Verification items for this drawing (mm, ordinates from the low corner). Round coordinates to 2 decimals unless told otherwise and drop trailing zeros. Write each loop counter-clockwise with the first axis right and the second up, starting at its lowest first coordinate (ties: lowest second). Pieces come first, ordered by that corner, then holes. Notation, with made-up numbers: (61, 12) -> (86, 12) arc R10 cw to (86, 26) -> close; hole circle Ø8 at (3.5, 79). An arc over 180 degrees is marked (long way). One line per question, with ' | ' between items.
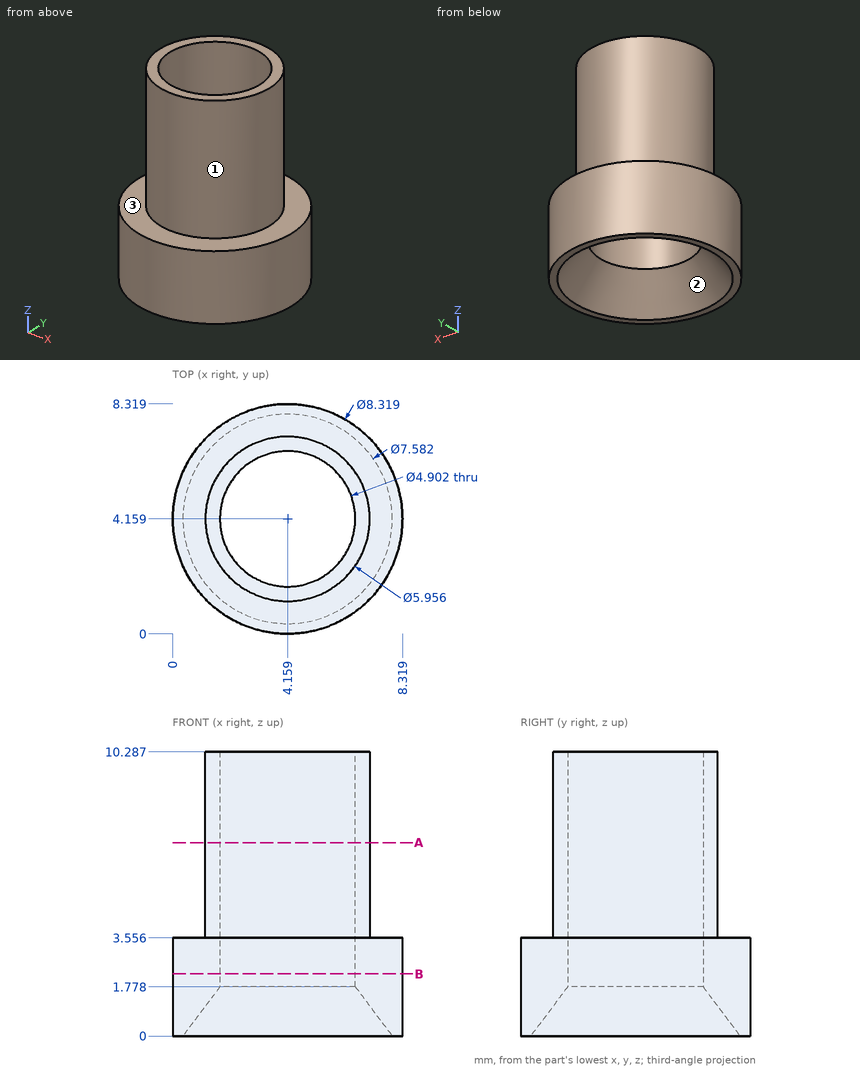
(1) Sectioned sample at B-B on z = 2.25. Record the cut outline in (x, y).
Resolved:
outline: circle Ø8.32 at (4.16, 4.16); hole circle Ø4.9 at (4.16, 4.16)
(2) Draft check along X on the marked faces 1, 2 and 3. Enter one of: +X half, -X half, draft (parallel to the pull), parting line (faces both ways), or undercut.
Resolved:
face 1: parting line | face 2: undercut | face 3: draft
(3) Material ranges on line 1 (Y direction, x = 4.25, z = 6) (1 decimal); line 2 (Z direction, x = 1, y = 1.5) (1 decimal); line 3 (X direction, y = 2.25, z = 0.75) (1 decimal), recorded low to high.
Resolved:
line 1: y = 1.2 to 1.7, 6.6 to 7.1 | line 2: z = 0 to 3.6 | line 3: x = 0.5 to 1.6, 6.8 to 7.9
(4) Go/stop test with flat-tipped pins: pin 1 (2 mm diameter, centred on y = 3, z = 9, fed in from -X) (1 decimal); pin 2 (4 mm diameter, centred on y = 1, z = 6, fed in from +X); pin 3 (1 mm diameter, centred on x = 2.5, z = 9, fed in from +Y). Record where each tip stops, or that it passes through.
Resolved:
pin 1: stops at x = 1.2 | pin 2: stops at x = 6.9 | pin 3: stops at y = 6.9
(5) Sectioned sample at A-A on z = 7. Record the cut outline in (x, y).
Resolved:
outline: circle Ø5.96 at (4.16, 4.16); hole circle Ø4.9 at (4.16, 4.16)
